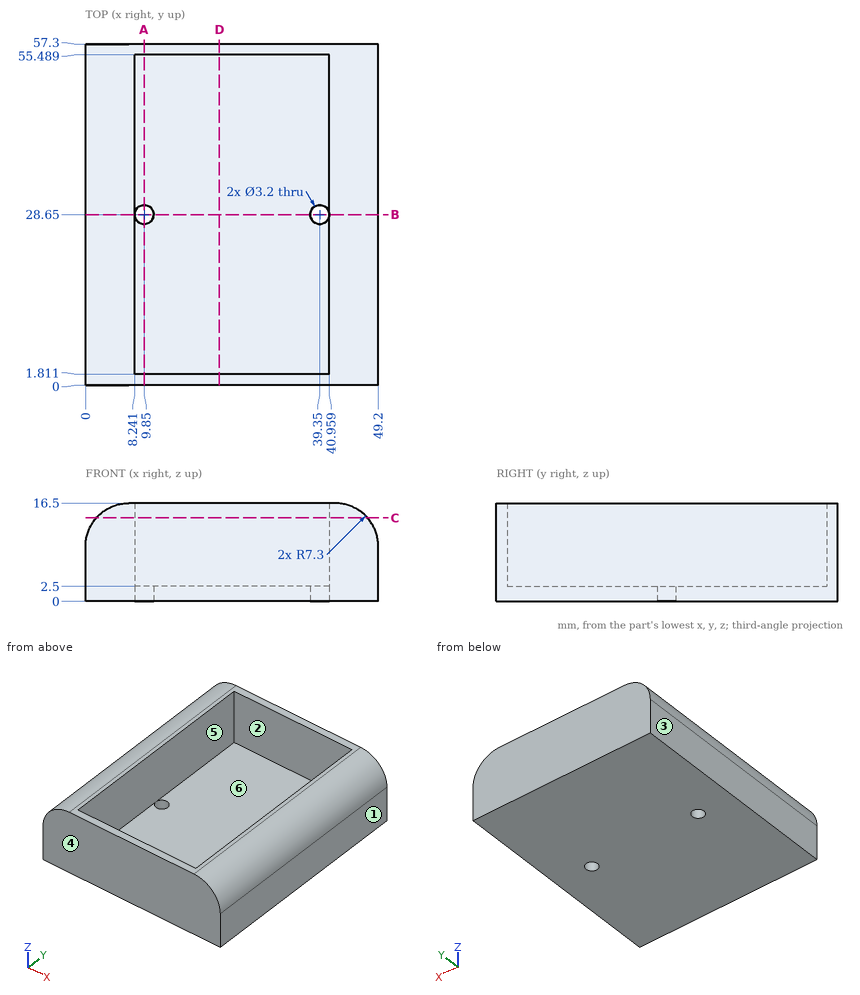
Input: dimensioned drawing with shaded views. Units: mm. Origin: part minimum x, y, z. A direction names the side the tool comes from. Give positions to 0.01 mm unless a question says otherwise; leave off trailing zeros. Write each loop counter-clockwise with the first axis right and the second up, starting at its lowest first coordinate (ties: lowest second). Pieces come first, ordered by that corner, then holes. Notation, with made-up numbers: M 80.5,65.5 L 105.5,65.5 A25 cw 105.5,93.5 Z; hole C -0.75,70 d7. An arc over 180 degrees is marked long. Write item = value, one per line. Start each with the question number.
1) First-contact query: pin 1 Ø4 at (y, z) = (22.5, 12) entering from +X; pin 2 Ø6 at (y, z) = (49, 13.5) entering from +X. Flat tips, straight axial feed; report the tip coordinate or a pass-through.
2) Material intervals for line 1 along X through (y, z) = (28.65, 2); line 2 along X through (y, z) = (42.5, 6); line 3 along Y through (x, z) = (15.5, 15.5), sorted ascending. Write a range as [from, to].
3) Cut plane C-C on z = 14. Return the cut outline in (x, y), then the cut area to 3 significant figures.
4) Cut plane D-D on x = 22.5. Return the cut outline in (y, z).
5) Cut plane A-A on x = 9.85. Return the cut outline in (y, z), then the cut area to 3 significant figures.
6) Reachability of the marked faces 1 and 2 from +Z, -Z, +X, -X, +Y, -Y: full face, straight path, thin tool, end or side. Return the list, or none.
7) Cut plane B-B on y = 28.65. Count the separate pieces of the cut face and the enclosed holes in it, then the cut area to 3 significant figures.
8) Draft query along X for the marked faces 3, 4, 5 and 6. Return one class per face: +X half, -X half, draft (parallel to the pull), parting line (faces both ways), or undercut.
Solved:
q1.pin_1 = 49.16
q1.pin_2 = 49.08
q2.line_1 = [0, 8.25], [11.45, 37.75], [40.95, 49.2]
q2.line_2 = [0, 8.24], [40.96, 49.2]
q2.line_3 = [0, 1.81], [55.49, 57.3]
q3.outline = M 1.8,0 L 47.4,0 L 47.4,57.3 L 1.8,57.3 Z; hole M 8.24,1.81 L 40.96,1.81 L 40.96,55.49 L 8.24,55.49 Z
q3.area = 857 mm2
q4.outline = M 0,0 L 57.3,0 L 57.3,16.5 L 55.49,16.5 L 55.49,2.5 L 1.81,2.5 L 1.81,16.5 L 0,16.5 Z
q5.outline = M 0,0 L 27.05,0 L 27.05,2.5 L 1.81,2.5 L 1.81,16.5 L 0,16.5 Z; M 30.25,0 L 57.3,0 L 57.3,16.5 L 55.49,16.5 L 55.49,2.5 L 30.25,2.5 Z
q5.area = 186 mm2
q6.face_1 = +Z, -Z, +X, +Y, -Y
q6.face_2 = +Z
q7.separate_pieces = 3
q7.enclosed_holes = 0
q7.area = 315 mm2
q8.face_3 = -X half
q8.face_4 = draft
q8.face_5 = undercut
q8.face_6 = undercut
